For this review, take the finished solid that the model builds, in its own axes (mm). A direction names the side the tool comes from. Give positions to 0.01 mm unless a question says otherwise; leave off trailing zeros. Loops run counter-clockwise (first coordinate to the right, second up) from the corner with the lowest first, then second, coordinate; pieces in that order, holes last. Notation, with made-up numbers: (59, 71.5) -> (113, 71.5) arc R31 ccw to (113, 103.5) -> close; hole circle Ø2 at (62.25, 27.25). An arc over 180 degrees is marked (long way). Write each question's results on one line, items separated by ' | '. Start each with the question number.
```python
from build123d import *

# Parameters (mm, degrees)
SALIENTE_EXTRUIR1_DEPTH = 40
CROQUIS5_R              = 1.45
CORTAR_EXTRUIR3_DEPTH   = 15
CROQUIS6_R              = 4
CORTAR_EXTRUIR4_DEPTH   = 106
CROQUIS8_R              = 10.1
CORTAR_EXTRUIR5_DEPTH   = 27
CROQUIS9_R              = 3.75
CORTAR_EXTRUIR6_DEPTH   = 80
CROQUIS12_R             = 1.5
CORTAR_EXTRUIR8_DEPTH   = 15
CROQUIS16_W             = 80
CROQUIS16_H             = 3
CORTAR_EXTRUIR11_DEPTH  = 80
CROQUIS21_R             = 33
CROQUIS21_R_2           = 22.4
CORTAR_EXTRUIR12_DEPTH  = 1
SALIENTE_EXTRUIR2_START = 2.5
CROQUIS22_R             = 22.4
SALIENTE_EXTRUIR2_DEPTH = 2.5
SALIENTE_EXTRUIR3_START = 1.5
CROQUIS24_R             = 40
CROQUIS24_R_2           = 33
SALIENTE_EXTRUIR3_DEPTH = 1.5
CROQUIS25_R             = 13
CORTAR_EXTRUIR13_DEPTH  = 7
CROQUIS26_R             = 9
CORTAR_EXTRUIR14_DEPTH  = 24
CORTAR_EXTRUIR15_START  = -25.5
CROQUIS27_R             = 9
CORTAR_EXTRUIR15_DEPTH  = 25.5
CROQUIS28_R             = 45
CROQUIS28_R_2           = 40
CORTAR_EXTRUIR16_DEPTH  = 25


with BuildPart() as part:
    # Croquis1 → Saliente-Extruir1 (new body)
    with BuildSketch(Plane(origin=(0, 0, 0), x_dir=(1, 0, 0), z_dir=(0, 1, 0))):
        with BuildLine():
            ThreePointArc((-40, -20.615528128), (-31.819805153, -31.819805153), (-20.615528128, -40))
            Line((-20.615528128, -40), (20.615528128, -40))
            ThreePointArc((20.615528128, -40), (31.819805153, -31.819805153), (40, -20.615528128))
            Line((40, -20.615528128), (40, 20.615528128))
            ThreePointArc((40, 20.615528128), (31.819805153, 31.819805153), (20.615528128, 40))
            Line((20.615528128, 40), (-20.615528128, 40))
            ThreePointArc((-20.615528128, 40), (-31.819805153, 31.819805153), (-40, 20.615528128))
            Line((-40, 20.615528128), (-40, -20.615528128))
        make_face()
    extrude(amount=SALIENTE_EXTRUIR1_DEPTH)

    # Croquis5 → Cortar-Extruir3 (cut)
    with BuildSketch(Plane(origin=(0, 40, 0), x_dir=(1, 0, 0), z_dir=(0, 1, 0))):
        with Locations(Location((-34.5, 14.446020213, 0), (0, 0, 270))):
            Circle(CROQUIS5_R)
        with Locations(Location((-34.5, -14.446020213, 0), (0, 0, 270))):
            Circle(CROQUIS5_R)
        with Locations(Location((-34.5, 0, 0), (0, 0, 270))):
            Circle(CROQUIS5_R)
    cortar_extruir3 = extrude(amount=-CORTAR_EXTRUIR3_DEPTH, mode=Mode.SUBTRACT)

    # Simetría1: Cortar-Extruir3 across plane
    add(cortar_extruir3.mirror(Plane(origin=(0, 0, 0), x_dir=(0, 0, 1), z_dir=(1, 0, 0))), mode=Mode.SUBTRACT)

    # Croquis6 → Cortar-Extruir4 (cut)
    with BuildSketch(Plane.XY.offset(40)):
        with Locations((-10, 40)):
            Circle(CROQUIS6_R)
        with Locations((10, 40)):
            Circle(CROQUIS6_R)
    extrude(amount=-CORTAR_EXTRUIR4_DEPTH, mode=Mode.SUBTRACT)

    # Croquis8 → Cortar-Extruir5 (cut)
    with BuildSketch(Plane.XZ):
        with Locations(Location((0, 0, 0), (0, 0, 270))):
            Circle(CROQUIS8_R)
    extrude(amount=-CORTAR_EXTRUIR5_DEPTH, mode=Mode.SUBTRACT)

    # Croquis9 → Cortar-Extruir6 (cut)
    with BuildSketch(Plane.ZY.offset(40)):
        with Locations((0, 14)):
            Circle(CROQUIS9_R)
    extrude(amount=-CORTAR_EXTRUIR6_DEPTH, mode=Mode.SUBTRACT)

    # Croquis12 → Cortar-Extruir8 (cut)
    with BuildSketch(Plane(origin=(0, 40, 0), x_dir=(1, 0, 0), z_dir=(0, 1, 0))):
        with Locations(Location((-16.875, 30, 0), (0, 0, 270))):
            Circle(CROQUIS12_R)
        with Locations(Location((0, 30, 0), (0, 0, 270))):
            Circle(CROQUIS12_R)
        with Locations(Location((16.875, 30, 0), (0, 0, 270))):
            Circle(CROQUIS12_R)
        with Locations(Location((-16.875, -30, 0), (0, 0, 270))):
            Circle(CROQUIS12_R)
        with Locations(Location((0, -30, 0), (0, 0, 270))):
            Circle(CROQUIS12_R)
        with Locations(Location((16.875, -30, 0), (0, 0, 270))):
            Circle(CROQUIS12_R)
    extrude(amount=-CORTAR_EXTRUIR8_DEPTH, mode=Mode.SUBTRACT)

    # Croquis16 → Cortar-Extruir11 (cut)
    with BuildSketch(Plane(origin=(40, 0, 0), x_dir=(0, 0, -1), z_dir=(1, 0, 0))):
        with Locations((0, 1.5)):
            Rectangle(CROQUIS16_W, CROQUIS16_H)
    extrude(amount=-CORTAR_EXTRUIR11_DEPTH, mode=Mode.SUBTRACT)

    # Croquis21 → Cortar-Extruir12 (cut)
    with BuildSketch(Plane.XZ.offset(-3)):
        with Locations(Location((0, 0, 0), (0, 0, 270))):
            Circle(CROQUIS21_R)
        with Locations(Location((0, 0, 0), (0, 0, 270))):
            Circle(CROQUIS21_R_2, mode=Mode.SUBTRACT)
    extrude(amount=-CORTAR_EXTRUIR12_DEPTH, mode=Mode.SUBTRACT)

    # Croquis22 → Saliente-Extruir2 (add)
    with BuildSketch(Plane.XZ.offset(-3).offset(SALIENTE_EXTRUIR2_START)):
        with Locations(Location((0, 0, 0), (0, 0, 270))):
            Circle(CROQUIS22_R)
    extrude(amount=-SALIENTE_EXTRUIR2_DEPTH)

    # Croquis24 → Saliente-Extruir3 (add)
    with BuildSketch(Plane.XZ.offset(-3).offset(SALIENTE_EXTRUIR3_START)):
        with Locations(Location((0, 0, 0), (0, 0, 270))):
            Circle(CROQUIS24_R)
        with Locations(Location((0, 0, 0), (0, 0, 270))):
            Circle(CROQUIS24_R_2, mode=Mode.SUBTRACT)
    extrude(amount=-SALIENTE_EXTRUIR3_DEPTH)

    # Croquis25 → Cortar-Extruir13 (cut)
    with BuildSketch(Plane.XZ.offset(-0.5)):
        with Locations(Location((0, 0, 0), (0, 0, 270))):
            Circle(CROQUIS25_R)
    extrude(amount=-CORTAR_EXTRUIR13_DEPTH, mode=Mode.SUBTRACT)

    # Croquis26 → Cortar-Extruir14 (cut)
    with BuildSketch(Plane(origin=(40, 0, 0), x_dir=(0, 0, -1), z_dir=(1, 0, 0))):
        with Locations((0, 14)):
            Circle(CROQUIS26_R)
    extrude(amount=-CORTAR_EXTRUIR14_DEPTH, mode=Mode.SUBTRACT)

    # Croquis27 → Cortar-Extruir15 (cut)
    with BuildSketch(Plane.ZY.offset(40).offset(CORTAR_EXTRUIR15_START)):
        with Locations(Location((0, 14, 0), (0, 0, 180))):
            Circle(CROQUIS27_R)
    extrude(amount=CORTAR_EXTRUIR15_DEPTH, mode=Mode.SUBTRACT)

    # Croquis28 → Cortar-Extruir16 (cut)
    with BuildSketch(Plane.XZ.offset(-0.5)):
        Circle(CROQUIS28_R)
        with Locations(Location((0, 0, 0), (0, 0, 270))):
            Circle(CROQUIS28_R_2, mode=Mode.SUBTRACT)
    extrude(amount=-CORTAR_EXTRUIR16_DEPTH, mode=Mode.SUBTRACT)


solid = part.part
```
1. Machinability: for faces 4 (the flat face through (29, 25.5, 29)), 5 (the cylindrical face through (16.9, 32.6, -31.5)), 6 (the flat face through (-22, 4, -7)), which of the approach directions +Z, -Z, +X, -X, +Y, -Y give a long, thin tool a straight path to every point of the face, cutting with its end or side? Answer none if there is none.
2. Wall thickness on L1, parallel to X at y = 3, z = 0; L2, parallel to Z at x = 0.5, y = 2.5; L3, parallel to X at y = 34, z = 30 (3 decimals): over which ranges is each line inside the solid? List them lowest first.
3. For pin 1 Ø5 at (x, y) = (-30, 18) entering from +Z; pin 2 Ø6 at (y, z) = (18, 20) entering from +X; pin 3 Ø6 at (y, z) = (15, -0.5) entering from -X; pin 4 Ø4.5 at (y, z) = (14, 0) entering from -X, all flat-tipped, find the tip position at first contact; note any pin that passes through.
4. Draft analysis for pull direction Z (two halves, no side actions). For faces 1 (the cylindrical face through (16.9, 32.6, 28.5)), 2 (the flat face through (0, 33, 40)), 3 (the flat face through (-40, 33, 0)), state which applies: released by +Z, released by -Z, zero draft, split by the parting line, or undercut.
5. We need section B-B (x = -34.5). Write out the cut boundary in (y, z), plus the area to 3 significant figures.
6. We need section A-A (y = 14). Write out the cut boundary in (x, z).
7. We need section C-C (y = 29). Count the separate pieces of the cut face and the enclosed holes in it, plus the area to 3 significant figures.
8. We need section D-D (z = -26). Write out the cut boundary in (x, y).
Response:
1) face 4: +Z, +X, -Y | face 5: +Y | face 6: -Y
2) L1: x = -40 to -33, -22.4 to -13, 13 to 22.4, 33 to 40 | L2: z = -40 to -33, -22.39 to -12.99, 12.99 to 22.39, 33 to 40 | L3: x = -33.541 to -18.375, -15.375 to -1.5, 1.5 to 15.375, 18.375 to 33.541
3) pin 1: stops at z = 29.05 | pin 2: stops at x = 36.21 | pin 3: stops at x = -14.5 | pin 4: passes through
4) face 1: undercut | face 2: released by +Z | face 3: zero draft
5) outline: (1.5, -20.24) -> (25.5, -20.24) -> (25.5, -28.89) -> (40, -28.89) -> (40, -15.9) -> (25, -15.9) -> (25, -13) -> (40, -13) -> (40, -1.45) -> (25, -1.45) -> (25, 1.45) -> (40, 1.45) -> (40, 13) -> (25, 13) -> (25, 15.9) -> (40, 15.9) -> (40, 28.89) -> (25.5, 28.89) -> (25.5, 20.24) -> (1.5, 20.24) -> close; hole circle Ø18 at (14, 0) | area: 1,420 mm2
6) outline: (-38.97, -9) arc R40 ccw to (38.97, -9) -> (16, -9) -> (16, -3.75) -> (9.38, -3.75) arc R10.1 cw to (-9.38, -3.75) -> (-14.5, -3.75) -> (-14.5, -9) -> close; (-38.97, 9) -> (-14.5, 9) -> (-14.5, 3.75) -> (-9.38, 3.75) arc R10.1 cw to (9.38, 3.75) -> (16, 3.75) -> (16, 9) -> (38.97, 9) arc R40 ccw to start
7) separate pieces: 1 | enclosed holes: 12 | area: 5,720 mm2
8) outline: (-36.73, 25.5) -> (-30.4, 25.5) -> (-30.4, 1.5) -> (-20.32, 1.5) -> (-20.32, 4) -> (20.32, 4) -> (20.32, 1.5) -> (30.4, 1.5) -> (30.4, 25.5) -> (36.73, 25.5) -> (36.73, 40) -> (14, 40) arc R4 cw to (6, 40) -> (-6, 40) arc R4 cw to (-14, 40) -> (-36.73, 40) -> close
